```python
from build123d import *

# Parameters (mm, degrees)
SKETCH_R  = 2.9
PAD_DEPTH = 3.5


with BuildPart() as part:
    # Sketch → Pad (new body)
    with BuildSketch(Plane.XY):
        Polygon((0, -10), (0, 15.091605), (40.351065, 60.700187), (72.199177, -10), align=None)
        with Locations((21.815896, 24.658385)):
            Circle(SKETCH_R, mode=Mode.SUBTRACT)
        with Locations((38.381398, 43.382278)):
            Circle(SKETCH_R, mode=Mode.SUBTRACT)
        with Locations((60, 0)):
            Circle(SKETCH_R, mode=Mode.SUBTRACT)
        with Locations((35, 0)):
            Circle(SKETCH_R, mode=Mode.SUBTRACT)
        with Locations((10, 0)):
            Circle(SKETCH_R, mode=Mode.SUBTRACT)
    extrude(amount=PAD_DEPTH)


solid = part.part
```
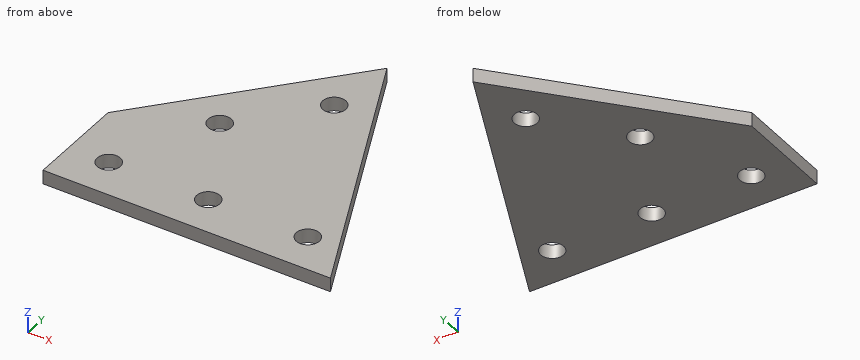
CAD build for the part. Positions are in the model's coordinates, mm. Round coordinates to 2 decimals unless told otherwise and drop trailing zeros. Loops run counter-clockwise (first coordinate to the right, second up) from the corner with the lowest first, then second, coordinate; pieces in that order, holes last. Notation, with made-up numbers: (13, 31) - (44, 31) arc R24 cw to (44, 48) - close; hole circle Ø5 at (35, -25). An arc over 180 degrees is marked (long way). Return JSON: item names as keys, results as strings. Group by question number.
Q1. Band-saw the part on B-B on z = 2.7. Give the cut face in (x, y).
Q2. Drill centre lines: line 1 along X through (y, z) = (2.5, 2.05); line 2 along X through (y, z) = (-1.5, 0.5); line 3 along Y through (x, z) = (38.5, 2.7). Where is each one in solid material? Low to high. Write a range as [from, to].
Q3. Band-saw the part on C-C on x = 9.5. Give the cut face in (y, z).
Q4. Band-saw the part on A-A on y = 1.5. Give the cut face in (x, z), plus the area to 3 significant figures.
Q5. Band-saw the part on D-D on y = 51. Give the cut face in (x, z), plus the area to 3 significant figures.
Q6. Flat gauge pins, fed straight in: pin 1 Ø1.5 at (y, z) = (41.5, 2) entering from -X; pin 2 Ø5 at (x, y) = (21.82, 24.66) entering from +Z. Where does each tip first touch, or does it go through?
Solutions:
{
 "1": {"outline": "(0, -10) - (72.2, -10) - (40.35, 60.7) - (0, 15.09) - close; hole circle Ø5.8 at (10, 0); hole circle Ø5.8 at (21.82, 24.66); hole circle Ø5.8 at (35, 0); hole circle Ø5.8 at (38.38, 43.38); hole circle Ø5.8 at (60, 0)"},
 "2": {"line 1": "x = [0, 8.53], [11.47, 33.53], [36.47, 58.53], [61.47, 66.57]", "line 2": "x = [0, 7.52], [12.48, 32.52], [37.48, 57.52], [62.48, 68.37]", "line 3": "y = [-10, 40.48], [46.28, 58.61]"},
 "3": {"outline": "(-10, 0) - (-2.86, 0) - (-2.86, 3.5) - (-10, 3.5) - close; (2.86, 0) - (25.83, 0) - (25.83, 3.5) - (2.86, 3.5) - close"},
 "4": {"outline": "(0, 0) - (7.52, 0) - (7.52, 3.5) - (0, 3.5) - close; (12.48, 0) - (32.52, 0) - (32.52, 3.5) - (12.48, 3.5) - close; (37.48, 0) - (57.52, 0) - (57.52, 3.5) - (37.48, 3.5) - close; (62.48, 0) - (67.02, 0) - (67.02, 3.5) - (62.48, 3.5) - close", "area": "182 mm^2"},
 "5": {"outline": "(31.77, 0) - (44.72, 0) - (44.72, 3.5) - (31.77, 3.5) - close", "area": "45.3 mm^2"},
 "6": {"pin 1": "stops at x = 22.7", "pin 2": "passes through"}
}
